Design review of the part shown in the three views and the two pictorial views. Dimensions are in mm from the part's minimum x, y and z. A direction names the side the tool comes from. Round coordinates to 2 decimals unless told otherwise and drop trailing zeros. Order: outer loops, then holes, each group sorted by start corner. A loop starts at its lowest first (then second) coordinate and runs counter-clockwise, first axis right, second up.
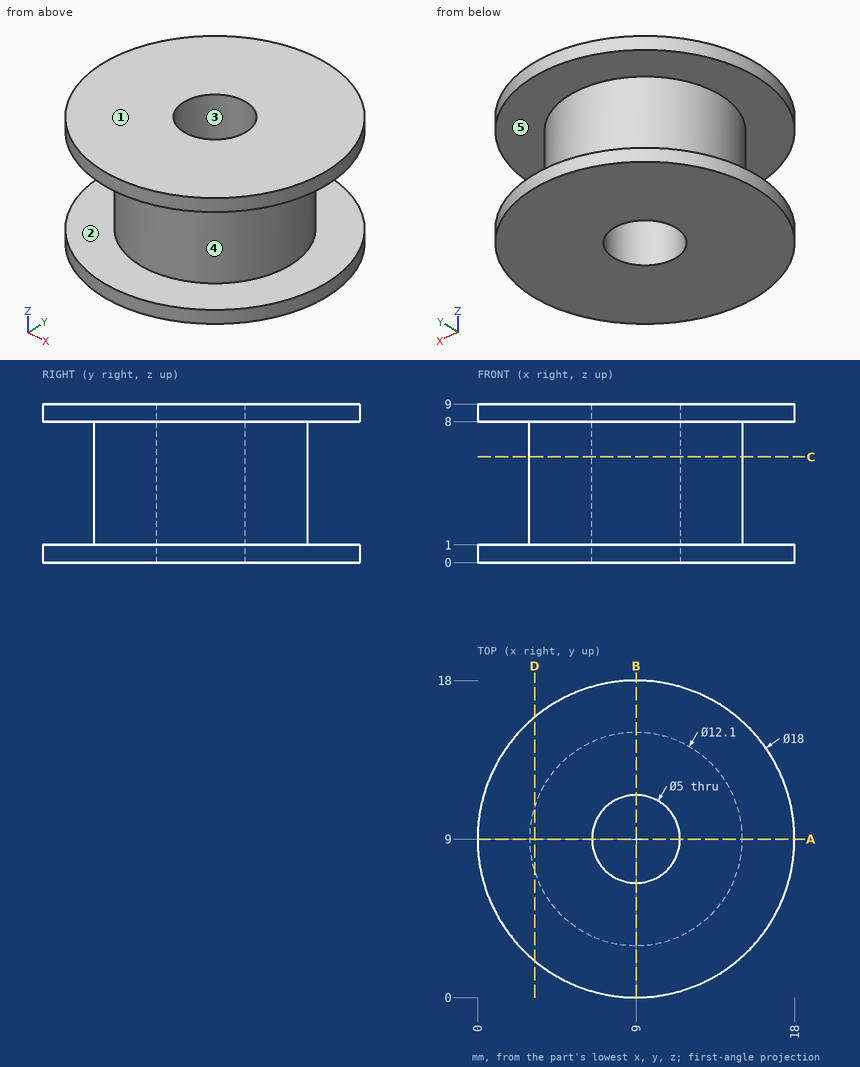
(1) Draft analysis for pull direction Y (two halves, no side actions). For the marked faces 3, 4 and 5, state which applies: pulls with the +Y half, pulls with the -Y half, needs draft (parallel to the pull), parting line crosses it, or undercut.
(2) Add section A-A on y = 9. Give the boundary of the cut face in (x, z), plus the area to 3 significant figures.
(3) Clearance check with flat-ended pins moving along their axes: P1, Ø1, axis at x = 4.5, z = 3, coming from the +Y side; P2, Ø2, axis at y = 15.5, z = 6, coming from the -X side; P3, Ø2, axis at y = 10.5, z = 6, coming from the +X side. State where each tip first meets the part, or that it passes through.
(4) Tool access review of the marked faces 1 and 2: name each direction out of +Z, -Z, +X, -X, +Y, -Y from which nothing blocks a thin tool from reaching the whole face with its end or side.
(5) Wall thickness on L1, parallel to Z at x = 16.75, y = 13.25; L2, parallel to Y at x = 9, z = 7.25; L3, parallel to Y at x = 7.75, z = 4.5: over which ranges is each line inside the solid? List them lowest first.
(6) Add section C-C on z = 6. Give the boundary of the cut face in (x, y).
(7) Add section D-D on x = 3.25. Give the boundary of the cut face in (y, z), plus the area to 3 significant figures.
Here are the results:
1. face 3: undercut
1. face 4: parting line crosses it
1. face 5: needs draft
2. outline: (0, 0) - (6.5, 0) - (6.5, 9) - (0, 9) - (0, 8) - (2.95, 8) - (2.95, 1) - (0, 1) - close; (11.5, 0) - (18, 0) - (18, 1) - (15.05, 1) - (15.05, 8) - (18, 8) - (18, 9) - (11.5, 9) - close
2. area: 75.7 mm2
3. P1: stops at y = 13.54
3. P2: stops at x = 6.48
3. P3: stops at x = 15.03
4. face 1: +Z, +X, -X, +Y, -Y
4. face 2: none
5. L1: z = 0 to 1, 8 to 9
5. L2: y = 2.95 to 6.5, 11.5 to 15.05
5. L3: y = 3.08 to 6.83, 11.17 to 14.92
6. outline: circle Ø12.1 at (9, 9); hole circle Ø5 at (9, 9)
7. outline: (2.08, 0) - (15.92, 0) - (15.92, 1) - (10.88, 1) - (10.88, 8) - (15.92, 8) - (15.92, 9) - (2.08, 9) - (2.08, 8) - (7.12, 8) - (7.12, 1) - (2.08, 1) - close
7. area: 54.0 mm2
